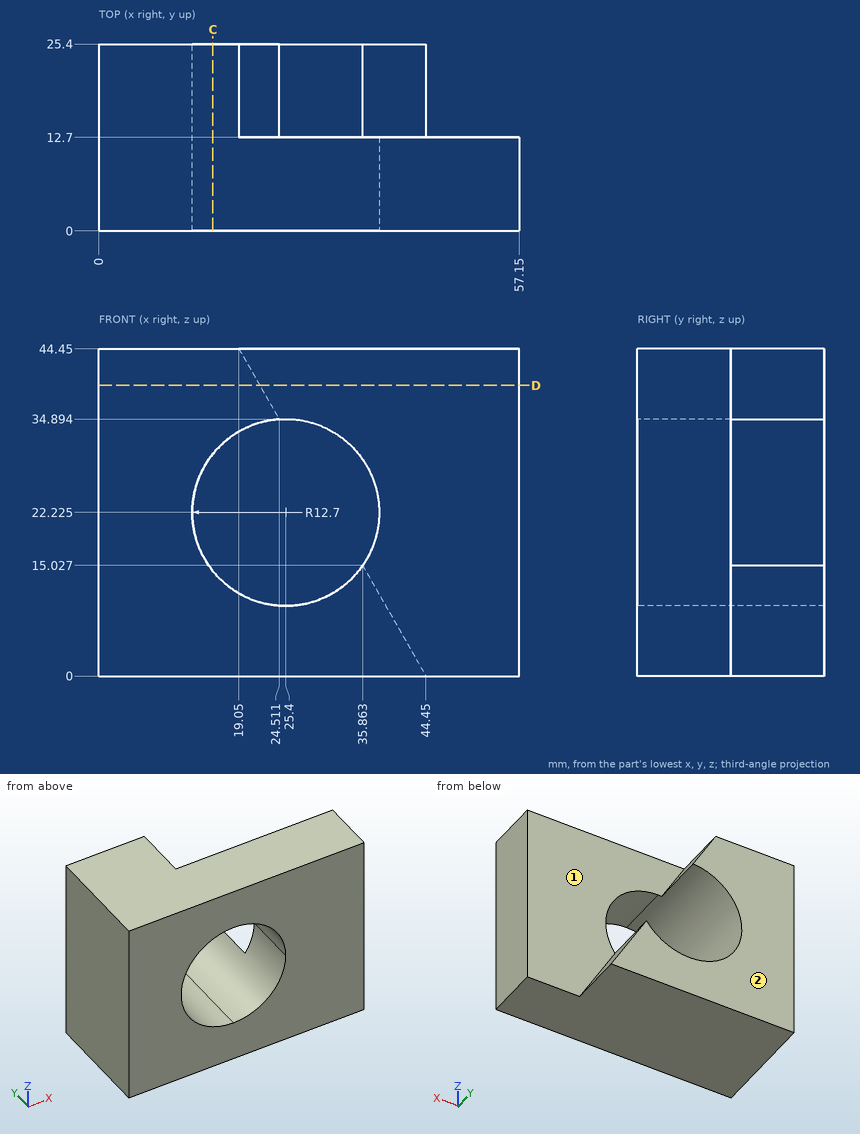
Check sheet for the drawn part. Datum: minimum x, y, z corner. Units: mm. A direction names the side the tool comes from. Give positions to 0.01 mm unless a question says otherwise; leave off trailing zeros. Write each loop counter-clockwise with the first axis right and the second up, starting at its lowest first coordinate (ties: lowest second). Pieces come first, ordered by that corner, then holes. Notation, with made-up numbers: M 77,78.25 L 122,78.25 A31 cw 122,102.25 Z; hole C 74,25 d10. An arc over 180 degrees is marked long. One line per question, with ' | ' between items.
1) Gauge pin test, flat end, axial feed: pin 1 Ø3 at (x, z) = (45.5, 33.5) entering from +Y. Record the tip position at first contact, or that the pin passes through.
Result:
pin 1: stops at y = 12.7
2) Section check C-C on x = 15.5. Enter the section's corners in (y, z), plus the area to 3 significant figures.
Result:
outline: M 0,0 L 25.4,0 L 25.4,14.27 L 0,14.27 Z; M 0,30.18 L 25.4,30.18 L 25.4,44.45 L 0,44.45 Z | area: 725 mm2
3) Thickness scan on line 1 along Y through (x, z) = (53, 5); line 2 along Z through (x, y) = (21, 15.5) (1 decimal); line 3 along X through (y, z) = (7, 23). Record the ranges inside material, lowest first. Write a range as [from, to].
Result:
line 1: y = [0, 12.7] | line 2: z = [0, 10.3], [34.1, 41] | line 3: x = [0, 12.72], [38.08, 57.15]
4) Section check D-D on z = 39.5. Enter the section's corners in (x, y), plus the area to 3 significant figures.
Result:
outline: M 0,0 L 57.15,0 L 57.15,12.7 L 21.88,12.7 L 21.88,25.4 L 0,25.4 Z | area: 1,000 mm2
5) Set-up check for the marked faces 1 and 2: record each of +Z, -Z, +X, -X, +Y, -Y from which the full face is reachable in a straight line by a thin tool's end or side.
Result:
face 1: +Z, +X, +Y | face 2: +Z, -Z, +X, -X, +Y
